from build123d import *

# Parameters (mm, degrees)
SKETCH1_W           = 76.2
SKETCH1_H           = 101.6
BOSS_EXTRUDE1_DEPTH = 5.08
SKETCH4_W           = 76.2
SKETCH4_H           = 101.6
SKETCH4_W_2         = 69.85
SKETCH4_H_2         = 95.25
BOSS_EXTRUDE3_DEPTH = 6.35
SKETCH5_R           = 3.81
SKETCH5_R_2         = 2.54
BOSS_EXTRUDE4_DEPTH = 73.025
SKETCH6_R           = 2.54
CUT_EXTRUDE2_DEPTH  = 128.513312638
SKETCH7_W           = 44.45
SKETCH7_H           = 95.25
CUT_EXTRUDE3_DEPTH  = 128.158650905
FILLET1_R           = 1.27
SKETCH8_W           = 6.35
SKETCH8_H           = 12.7
BOSS_EXTRUDE5_DEPTH = 3.175
CHAMFER1_SIZE       = 3.175


with BuildPart() as part:
    # Sketch1 → Boss-Extrude1 (new body)
    with BuildSketch(Plane(origin=(0, 0, 0), x_dir=(1, 0, 0), z_dir=(0, 1, 0))):
        with Locations((38.1, 50.8)):
            Rectangle(SKETCH1_W, SKETCH1_H)
    extrude(amount=BOSS_EXTRUDE1_DEPTH)

    # Sketch4 → Boss-Extrude3 (add)
    with BuildSketch(Plane(origin=(0, 5.08, 0), x_dir=(1, 0, 0), z_dir=(0, 1, 0))):
        with Locations((38.1, 50.8)):
            Rectangle(SKETCH4_W, SKETCH4_H)
        with Locations((38.1, 50.8)):
            Rectangle(SKETCH4_W_2, SKETCH4_H_2, mode=Mode.SUBTRACT)
    extrude(amount=BOSS_EXTRUDE3_DEPTH)

    # Sketch5 → Boss-Extrude4 (add)
    # profile 1 of 2: a face of its own
    with BuildSketch(Plane(origin=(76.2, 0, 0), x_dir=(0, 0, -1), z_dir=(1, 0, 0))):
        with Locations((12.7, 7.62)):
            Circle(SKETCH5_R)
        with Locations((12.7, 7.62)):
            Circle(SKETCH5_R_2, mode=Mode.SUBTRACT)
    # profile 2 of 2: a face of its own
    with BuildSketch(Plane(origin=(76.2, 0, 0), x_dir=(0, 0, -1), z_dir=(1, 0, 0))):
        with Locations((88.9, 7.62)):
            Circle(SKETCH5_R)
        with Locations((88.9, 7.62)):
            Circle(SKETCH5_R_2, mode=Mode.SUBTRACT)
    extrude(amount=-BOSS_EXTRUDE4_DEPTH)

    # Sketch6 → Cut-Extrude2 (cut, through all)
    with BuildSketch(Plane(origin=(76.2, 0, 0), x_dir=(0, 0, -1), z_dir=(1, 0, 0))):
        with Locations((12.7, 7.62)):
            Circle(SKETCH6_R)
        with Locations((88.9, 7.62)):
            Circle(SKETCH6_R)
    extrude(amount=-CUT_EXTRUDE2_DEPTH, mode=Mode.SUBTRACT)

    # Sketch7 → Cut-Extrude3 (cut, through all)
    with BuildSketch(Plane(origin=(0, 5.08, 0), x_dir=(1, 0, 0), z_dir=(0, 1, 0))):
        with Locations((38.1, 50.8)):
            Rectangle(SKETCH7_W, SKETCH7_H)
    extrude(amount=CUT_EXTRUDE3_DEPTH, mode=Mode.SUBTRACT)

    # Fillet1
    fillet1_edges = [part.edges().sort_by_distance(p)[0] for p in [
        (66.675, 5.08, -91.739806331),
        (9.525, 5.08, -86.060193669),
        (66.675, 5.08, -15.539806331),
        (9.525, 5.08, -9.860193669),
        (66.675, 5.08, -9.860193669),
        (9.525, 5.08, -15.539806331),
        (66.675, 5.08, -86.060193669),
        (9.525, 5.08, -91.739806331),
    ]]
    fillet(fillet1_edges, radius=FILLET1_R)

    # Sketch8 → Boss-Extrude5 (add)
    with BuildSketch(Plane.XZ):
        with Locations((73.025, -6.35)):
            Rectangle(SKETCH8_W, SKETCH8_H)
        with Locations((73.025, -95.25)):
            Rectangle(SKETCH8_W, SKETCH8_H)
        with Locations((3.175, -95.25)):
            Rectangle(SKETCH8_W, SKETCH8_H)
        with Locations((3.175, -6.35)):
            Rectangle(SKETCH8_W, SKETCH8_H)
    extrude(amount=BOSS_EXTRUDE5_DEPTH)

    # Chamfer1
    chamfer1_edges = [part.edges().sort_by_distance(p)[0] for p in [
        (69.85, 0, -95.25),
        (73.025, 0, -88.9),
        (69.85, 0, -6.35),
        (73.025, 0, -12.7),
        (3.175, 0, -12.7),
        (6.35, 0, -6.35),
        (3.175, 0, -88.9),
        (6.35, 0, -95.25),
    ]]
    chamfer(chamfer1_edges, length=CHAMFER1_SIZE - 0.0001)  # a hair under: the kernel refuses the full size


solid = part.part
Could you check a few things on this model? Use its own coordinates, in mm. A direction names the side the tool comes from. Round coordinates to 2 decimals unless told otherwise and drop trailing zeros. Loops run counter-clockwise (first coordinate to the right, second up) from the corner with the lowest first, then second, coordinate; pieces in that order, holes last. Notation, with made-up numbers: (-39, -8) - (20, -8) arc R21 cw to (20, 6) - close; hole circle Ø9 at (7, -23.5). An arc over 180 degrees is marked (long way). Write item = value, one per line.
1) If we mould it in two halves opening along Z, with no side actions, what happens to faces 5 (the flat face through (60.325, 10.4, -88.9)), 6 (the flat face through (3, -3.175, -6)), 7 (the flat face through (3.175, 8, -96)), 8 (the flat face through (38, 6, -101.6))? For each: pulls with the +Z half, pulls with the -Z half, needs draft (parallel to the pull), parting line crosses it, or undercut.
Computed:
face_5 = undercut
face_6 = needs draft
face_7 = undercut
face_8 = pulls with the -Z half
2) I need wall thicknesses on line 1 along Z through (x, y) = (72.25, 7.62) (3 decimals); line 2 along Y through (x, z) = (5, -12.7); line 3 along X through (y, z) = (7, -97) (3 decimals). Which ranges of each line are inside material? Lowest first, please. Write a range as from..to.
Computed:
line_1 = -101.6..-98.425, -92.71..-91.44, -86.36..-85.09, -16.51..-15.24, -10.16..-8.89, -3.175..0
line_2 = -3.17..5.08, 10.16..11.43
line_3 = 0..3.175, 73.025..76.2
3) Imagine slicing it at B-B (z = -55). Please give me the cut outline in (x, y) (3 decimals), and give its area (3 significant figures).
Computed:
outline = (0, 0) - (76.2, 0) - (76.2, 11.43) - (73.025, 11.43) - (73.025, 5.08) - (3.175, 5.08) - (3.175, 11.43) - (0, 11.43) - close
area = 427 mm2
4) Imagine slicing it at A-A (x = 34.5). Please give me the cut outline in (y, z) (3 decimals), and give its area (3 significant figures).
Computed:
outline = (0, -101.6) - (11.43, -101.6) - (11.43, -98.425) - (5.08, -98.425) - (5.08, -3.175) - (11.43, -3.175) - (11.43, 0) - (0, 0) - close
area = 556 mm2
5) I'm going to push a flat-ended pin straight in: P1, Ø8, axis at x = 24.5, z = -53.5, coming from the +Y side. Where does the tip first touch, or does it pass through?
Computed:
P1 = 5.08
6) On a 3-axis mill with a long thin cutter (end or side, diameter ignored), from which of +Z, -Z, +X, -X, +Y, -Y can I reach the whole of each face in a straight line? I mean faces 1 (the flat face through (3.637, -1.565, -14.31)), 2 (the cylindrical face through (66.76, 11.43, -12.8)), 3 (the flat face through (60.325, 9, -10)), 4 (the flat face through (7.96, -1.565, -8.049)). Say none if no direction works.
Computed:
face_1 = +X, -X, -Y
face_2 = none
face_3 = +Y
face_4 = +Z, -Z, -Y
